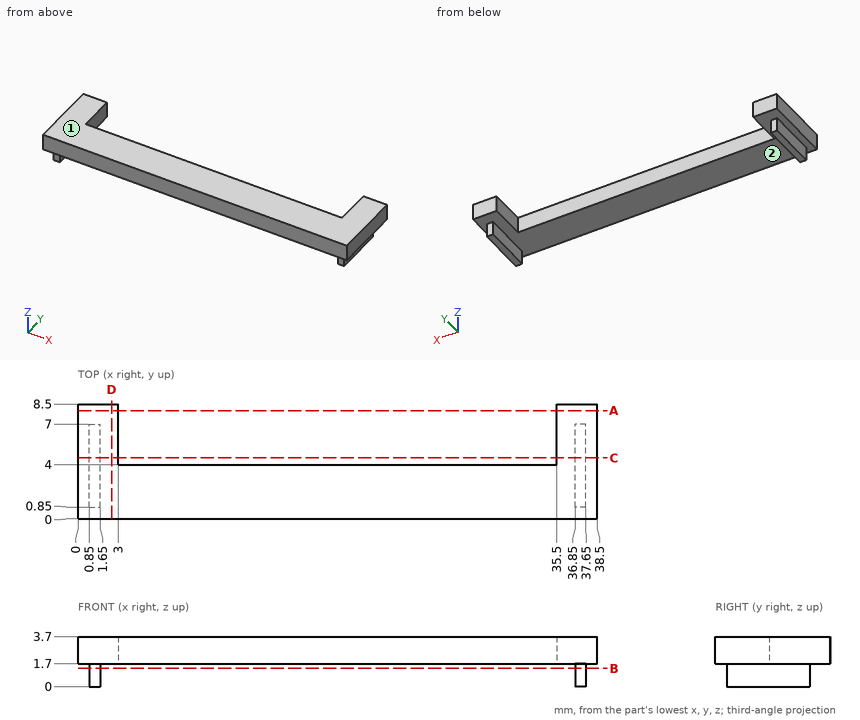
Here's the drawing with two shaded views (mm, measured from the low corner). I have some questions. Coordinates: 2 decimals unless noted, no trailing zeros. Order: outer loops, then holes, each group sorted by start corner. A loop starts at its lowest first (then second) coordinate and runs counter-clockwise, first axis right, second up.
Q1. Suppose I cut it at A-A on y = 8. Please give me the cut outline in (x, z), and give its area (3 significant figures).
Q2. Suppose I cut it at C-C on y = 4.5. Please give me the cut outline in (x, z), and give its area (3 significant figures).
Q3. Suppose I cut it at B-B on z = 1.35. Please give me the cut outline in (x, y), and give its area (3 significant figures).
Q4. Thinking about a two-plate mould opening in X: for the marked faces 1 and 2, which applies, released by +X, released by -X, zero draft, split by the parting line, or undercut?
Q5. Please list where these lines run through material, in increasing order: L1, parallel to X at y = 1.5, z = 0.5; L2, parallel to X at y = 7.5, z = 2.8; L3, parallel to Z at x = 25.5, y = 1.75.
Q6. Will these pins go through, and if not, where does the flat tip stop? pin 1 (0.9 mm diameter, centred on x = 1, z = 1, fed in from -Y); pin 2 (2 mm diameter, centred on x = 21.5, z = 3, fed in from +Y); pin 3 (1 mm diameter, centred on x = 30.5, y = 4, fed in from -Z).
Q7. Suppose I cut it at D-D on x = 2.5. Please give me the cut outline in (y, z), and give its area (3 significant figures).
Answer:
1. outline: (0, 1.7) - (3, 1.7) - (3, 3.7) - (0, 3.7) - close; (35.5, 1.7) - (38.5, 1.7) - (38.5, 3.7) - (35.5, 3.7) - close
1. area: 12.0 mm2
2. outline: (0, 1.7) - (0.85, 1.7) - (0.85, 0) - (1.65, 0) - (1.65, 1.7) - (3, 1.7) - (3, 3.7) - (0, 3.7) - close; (35.5, 1.7) - (36.85, 1.7) - (36.85, 0) - (37.65, 0) - (37.65, 1.7) - (38.5, 1.7) - (38.5, 3.7) - (35.5, 3.7) - close
2. area: 14.7 mm2
3. outline: (0.85, 0.85) - (1.65, 0.85) - (1.65, 7) - (0.85, 7) - close; (36.85, 0.85) - (37.65, 0.85) - (37.65, 7) - (36.85, 7) - close
3. area: 9.84 mm2
4. face 1: zero draft
4. face 2: undercut
5. L1: x = 0.85 to 1.65, 36.85 to 37.65
5. L2: x = 0 to 3, 35.5 to 38.5
5. L3: z = 1.7 to 3.7
6. pin 1: stops at y = 0.85
6. pin 2: stops at y = 4
6. pin 3: stops at z = 1.7
7. outline: (0, 1.7) - (8.5, 1.7) - (8.5, 3.7) - (0, 3.7) - close
7. area: 17.0 mm2
